```python
from build123d import *

# Parameters (mm, degrees)
F0_W     = 508
F0_H     = 228.6
F0_W_2   = 355.6
F0_H_2   = 53.975
F1_DEPTH = 9.525
F2_R     = 3.175


with BuildPart() as f1:
    # F0 (on Top) → F1 (new body, symmetric)
    with BuildSketch(Plane.XY):
        Rectangle(F0_W, F0_H)
        Rectangle(F0_W_2, F0_H_2, mode=Mode.SUBTRACT)
    extrude(amount=F1_DEPTH, both=True)

    # F2
    f2_edges = [f1.edges().sort_by_distance(p)[0] for p in [
        (-177.8, 0, 9.525),
        (0, 26.9875, 9.525),
        (0, -26.9875, 9.525),
        (177.8, 0, 9.525),
        (177.8, 26.9875, 0),
        (-177.8, 26.9875, 0),
        (-177.8, -26.9875, 0),
        (177.8, -26.9875, 0),
    ]]
    fillet(f2_edges, radius=F2_R)


solid = f1.part
```
For this review, take the finished solid that the model builds, in its own axes (mm). A direction names the side the tool comes from. Coordinates: 2 decimals unless noted, no trailing zeros. Write each loop counter-clockwise with the first axis right and the second up, starting at its lowest first coordinate (ties: lowest second). Pieces come first, ordered by that corner, then holes.
(1) Add section B-B on y = -18. Give the boundary of the cut face in (x, z) (3 decimals), then the cut area to 3 significant figures.
(2) Wall thickness on probe 1 along Y at (x, z) = (-28, 0.75); probe 2 along X at (y, z) = (9, -4); probe 3 along Y at (x, z) = (120.5, 9): over which ranges is each line inside the solid? List them lowest first.
(3) The part is to be moulded in two halves that separate along Y. For faces 3 (the face through (-4, 52, -9.525)), 4 (the face through (-2, 26.988, -1)), 5 (the face through (-4, -114.3, 0)), say which applies: +Y half, -Y half, draft (parallel to the pull), parting line (faces both ways), or undercut.
(4) Tool access review of faces 1 (the face through (177.8, 0, -1)), 2 (the face through (254, -2, 0)): name each direction out of +Z, -Z, +X, -X, +Y, -Y from which nothing blocks a thin tool from reaching the whole face with its end or side.
Answer sheet:
1. outline: (-254, -9.525) - (-177.8, -9.525) - (-177.8, 6.35) arc R3.175 ccw to (-180.975, 9.525) - (-254, 9.525) - close; (177.8, -9.525) - (254, -9.525) - (254, 9.525) - (180.975, 9.525) arc R3.175 ccw to (177.8, 6.35) - close
1. area: 2,900 mm2
2. probe 1: y = -114.3 to -26.99, 26.99 to 114.3
2. probe 2: x = -254 to -177.8, 177.8 to 254
2. probe 3: y = -114.3 to -28.41, 28.41 to 114.3
3. face 3: draft
3. face 4: undercut
3. face 5: -Y half
4. face 1: +Z, -Z
4. face 2: +Z, -Z, +X, +Y, -Y
